Can you work these out from the model? Positions are in its coordinate system, mm. A direction names the side the tool comes from. Coordinates: 2 decimals unless noted, no trailing zeros. Write each loop counter-clockwise with the first axis right and the second up, starting at its lowest first coordinate (ties: lowest second). Pieces come first, ordered by that corner, then holes. Notation, with made-up numbers: (31, 89.5) -> (65, 89.5) arc R29 cw to (65, 110.5) -> close; hole circle Ø3 at (59.25, 66). An arc over 180 degrees is marked (long way). Use one line per item in the form item = value.
```python
from build123d import *

# Parameters (mm, degrees)
F2_W     = 88.9
F2_H     = 35.9210244843
F3_DEPTH = 2.5
F4_R     = 5
F5_W     = 83.9
F5_H     = 30.9210244843
F5_W_2   = 79.9
F5_H_2   = 26.9210244843
F6_DEPTH = 4
F7_R     = 2.5
F8_R     = 2.49999
F9_R     = 0.5


# Not quite as in the source:
# - a fillet or chamfer is up to 0.001 mm smaller than in the source, because OpenCascade refuses the exact size


with BuildPart() as f3:
    # F2 (on Front) → F3 (new body)
    with BuildSketch(Plane.XZ):
        Rectangle(F2_W, F2_H)
    extrude(amount=-F3_DEPTH)

    # F4
    f4_edges = [f3.edges().sort_by_distance(p)[0] for p in [
        (44.45, 1.25, 17.960512),
        (44.45, 1.25, -17.960512),
        (-44.45, 1.25, -17.960512),
        (-44.45, 1.25, 17.960512),
    ]]
    fillet(f4_edges, radius=F4_R)

    # F5 (on Front) → F6 (join)
    with BuildSketch(Plane.XZ):
        Rectangle(F5_W, F5_H)
        Rectangle(F5_W_2, F5_H_2, mode=Mode.SUBTRACT)
    extrude(amount=F6_DEPTH)

    # F7
    f7_edges = [f3.edges().sort_by_distance(p)[0] for p in [
        (-41.95, -2, -15.460512),
        (-41.95, -2, 15.460512),
        (41.95, -2, -15.460512),
        (41.95, -2, 15.460512),
    ]]
    fillet(f7_edges, radius=F7_R)

    # F8 (radius 2.5 in the source; OpenCascade refuses exactly that, so slightly less here)
    f8_edges = [f3.edges().sort_by_distance(p)[0] for p in [
        (0, 2.5, -17.960512),
    ]]
    fillet(f8_edges, radius=F8_R)

    # F9
    f9_edges = [f3.edges().sort_by_distance(p)[0] for p in [
        (41.95, -4, 0),
    ]]
    fillet(f9_edges, radius=F9_R)


solid = f3.part
```
Q1. Suppose I cut it at A-A (y = -1.25). Write out the boundary of the cut face in (x, z).
Return value:
outline = (-41.95, -12.96) arc R2.5 ccw to (-39.45, -15.46) -> (39.45, -15.46) arc R2.5 ccw to (41.95, -12.96) -> (41.95, 12.96) arc R2.5 ccw to (39.45, 15.46) -> (-39.45, 15.46) arc R2.5 ccw to (-41.95, 12.96) -> close; hole (-39.95, -13.46) -> (39.95, -13.46) -> (39.95, 13.46) -> (-39.95, 13.46) -> close
Q2. For faces 1 (the cylindrical face through (41.237, -1.774, 14.709)), 2 (the flat face through (41.95, -2, 0)), 3 (the flat face through (-1, -2, 15.461)), which set-ups out of +Z, -Z, +X, -X, +Y, -Y let a thin tool reach every point of the face, with its end or its side?
Return value:
face_1 = +Z, +X, -Y
face_2 = +Z, -Z, +X, -Y
face_3 = +Z, +X, -X, -Y
Q3. If I drill on line 1 (Z direction, x = 9, y = -0.5); line 2 (X direction, y = -0.25, z = -5.5), over which ranges is the centre line in solid material (lowest first)? Write a range as from..to.
Return value:
line_1 = -15.46..-13.46, 13.46..15.46
line_2 = -41.95..-39.95, 39.95..41.95
Q4. Will these pins go through, and if not, where does the flat tip stop? pin 1 (2 mm diameter, centred on y = -2, z = 3, fed in from +X); pin 2 (11 mm diameter, centred on x = -19, z = 5, fed in from -Y); pin 3 (1.2 mm diameter, centred on x = -5.5, y = -1, fed in from +Z).
Return value:
pin_1 = 41.95
pin_2 = 0
pin_3 = 15.46
